Input: part model. Units: mm. Frame: model coordinates. Face numbers are marked on the shaded views. A direction names the side the tool comes from. Give positions to 0.01 mm unless a question says otherwise; leave off trailing zeros. Write each loop counter-clockwise with the first axis right and the second up, starting at its lowest first coordinate (ties: lowest second). Pieces come first, ordered by that corner, then holes.
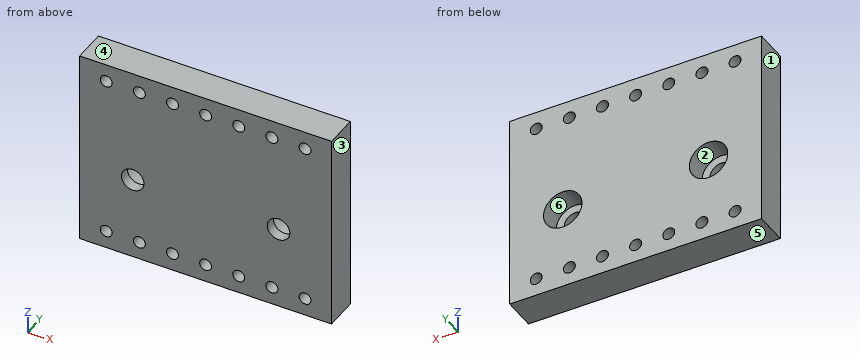
```python
from build123d import *

# Parameters (mm, degrees)
SKETCH1_W           = 48.26
SKETCH1_H           = 38.1
BOSS_EXTRUDE1_DEPTH = 6.35
SKETCH2_R           = 3.683
CUT_EXTRUDE1_DEPTH  = 4.318
SKETCH3_R           = 2.159
CUT_EXTRUDE2_DEPTH  = 4.318
SKETCH4_R           = 1.143
CUT_EXTRUDE3_DEPTH  = 9.398
LPATTERN1_COUNT     = 7
LPATTERN1_PITCH     = 6.35


with BuildPart() as part:
    # Sketch1 → Boss-Extrude1 (new body)
    with BuildSketch(Plane(origin=(0, 0, 0), x_dir=(1, 0, 0), z_dir=(0, 1, 0))):
        Rectangle(SKETCH1_W, SKETCH1_H)
    extrude(amount=-BOSS_EXTRUDE1_DEPTH)

    # Sketch2 → Cut-Extrude1 (cut)
    with BuildSketch(Plane(origin=(0, 0, 0), x_dir=(1, 0, 0), z_dir=(0, 1, 0))):
        with Locations((-13.97, 3.048)):
            Circle(SKETCH2_R)
    cut_extrude1 = extrude(amount=-CUT_EXTRUDE1_DEPTH, mode=Mode.SUBTRACT)

    # Sketch3 → Cut-Extrude2 (cut)
    with BuildSketch(Plane(origin=(0, -4.318, 0), x_dir=(1, 0, 0), z_dir=(0, 1, 0))):
        with Locations((-13.97, 3.048)):
            Circle(SKETCH3_R)
    cut_extrude2 = extrude(amount=-CUT_EXTRUDE2_DEPTH, mode=Mode.SUBTRACT)

    # Sketch4 → Cut-Extrude3 (cut)
    with BuildSketch(Plane(origin=(0, 0, 0), x_dir=(1, 0, 0), z_dir=(0, 1, 0))):
        with Locations((-19.05, 15.621)):
            Circle(SKETCH4_R)
        with Locations((-19.05, -15.621)):
            Circle(SKETCH4_R)
    cut_extrude3 = extrude(amount=-CUT_EXTRUDE3_DEPTH, mode=Mode.SUBTRACT)

    # LPattern1: Cut-Extrude3 ×7
    with Locations(*[(i * LPATTERN1_PITCH, 0, 0) for i in range(1, LPATTERN1_COUNT)]):
        add(cut_extrude3, mode=Mode.SUBTRACT)

    # Mirror1: Cut-Extrude1, Cut-Extrude2 across plane
    add(cut_extrude1.mirror(Plane(origin=(0, 0, 0), x_dir=(0, 0, 1), z_dir=(1, 0, 0))), mode=Mode.SUBTRACT)
    add(cut_extrude2.mirror(Plane(origin=(0, 0, 0), x_dir=(0, 0, 1), z_dir=(1, 0, 0))), mode=Mode.SUBTRACT)


solid = part.part
```
Q1. Section B-B, the plane y = -3.5. Give the number of separate pieces and of enclosed holes in the cut face, then the cut area to 3 significant figures.
Q2. Section A-A, the plane x = -6.35. Return the cut outline in (y, z).
Q3. Mould query, pull axis X, two halves, no side actions, for the marked faces 1, 2, 3 and 4. Classes: +X half, -X half, draft (parallel to the pull), parting line (faces both ways), or undercut.
Q4. Material intervals for line 1 along Z through (x, y) = (-19.05, -1.25); line 2 along X through (y, z) = (-3.25, -3); line 3 along Z through (x, y) = (12.5, -5.25), sorted ascending.
Q5. Section C-C, the plane x = -12.7. Return the cut outline in (y, z), then the cut area to 3 significant figures.
Q6. Pin query (flat end, axial travel): pin 1 (5 mm diameter, centred on x = -13.97, z = -3.048, fed in from -Y); pin 2 (2 mm diameter, centred on x = -12, z = -3, fed in from +Y). Return the tip coordinate at first contact, or that it passes through.
Q7. Access query for the marked faces 5 and 6. Directions: +Z, -Z, +X, -X, +Y, -Y. A direction counts if a zero-diameter tool reaches every point of the face in a straight line with its end or side. Return the directions, or none.
Q8. Section D-D, the plane z = 0. Return the cut outline in (x, y), then the cut area to 3 significant figures.
Solutions:
1. separate pieces: 1
1. enclosed holes: 16
1. area: 1,700 mm2
2. outline: (-6.35, -19.05) - (0, -19.05) - (0, -16.76) - (-6.35, -16.76) - close; (-6.35, -14.48) - (0, -14.48) - (0, 14.48) - (-6.35, 14.48) - close; (-6.35, 16.76) - (0, 16.76) - (0, 19.05) - (-6.35, 19.05) - close
3. face 1: -X half
3. face 2: undercut
3. face 3: +X half
3. face 4: draft
4. line 1: z = -19.05 to -16.76, -14.48 to 14.48, 16.76 to 19.05
4. line 2: x = -24.13 to -17.65, -10.29 to 10.29, 17.65 to 24.13
4. line 3: z = -19.05 to -16.75, -14.5 to -4.63, -1.47 to 14.5, 16.75 to 19.05
5. outline: (-6.35, -19.05) - (0, -19.05) - (0, -16.76) - (-6.35, -16.76) - close; (-6.35, -14.48) - (0, -14.48) - (0, -6.51) - (-4.32, -6.51) - (-4.32, -4.79) - (-6.35, -4.79) - close; (-6.35, -1.3) - (-4.32, -1.3) - (-4.32, 0.41) - (0, 0.41) - (0, 14.48) - (-6.35, 14.48) - close; (-6.35, 16.76) - (0, 16.76) - (0, 19.05) - (-6.35, 19.05) - close
5. area: 176 mm2
6. pin 1: stops at y = -6.35
6. pin 2: stops at y = -4.32
7. face 5: -Z, +X, -X, +Y, -Y
7. face 6: +Y
8. outline: (-24.13, -6.35) - (24.13, -6.35) - (24.13, 0) - (16.04, 0) - (16.04, -4.32) - (11.9, -4.32) - (11.9, 0) - (-11.9, 0) - (-11.9, -4.32) - (-16.04, -4.32) - (-16.04, 0) - (-24.13, 0) - close
8. area: 271 mm2
